from build123d import *

# Parameters (mm, degrees)
SKETCH1_W           = 103
SKETCH1_H           = 83.25
BOSS_EXTRUDE1_DEPTH = 20.2438
CUT_EXTRUDE1_DEPTH  = 17.2438
SKETCH3_W           = 15
SKETCH3_H           = 17.2438
SKETCH3_W_2         = 11
CUT_EXTRUDE2_DEPTH  = 14.9225
CUT_EXTRUDE3_DEPTH  = 2.4
SKETCH5_W           = 30
SKETCH5_H           = 6
BOSS_EXTRUDE2_DEPTH = 12.7
SKETCH6_W           = 30
SKETCH6_H           = 6
BOSS_EXTRUDE3_DEPTH = 12.7
FILLET1_R           = 4
FILLET2_R           = 0.5
FILLET3_R           = 2
FILLET4_R           = 4
FILLET5_R           = 2
SKETCH7_R           = 1.7145
CUT_EXTRUDE4_DEPTH  = 152.66642324
SKETCH8_R           = 3.81
CUT_EXTRUDE5_DEPTH  = 3.302
SKETCH11_R          = 2.38125
CUT_EXTRUDE7_DEPTH  = 151.98270874
CUT_EXTRUDE8_START  = -1
SKETCH12_R          = 4.699
CUT_EXTRUDE8_DEPTH  = 152.98270874


with BuildPart() as part:
    # Sketch1 → Boss-Extrude1 (new body)
    with BuildSketch(Plane(origin=(0, 0, 0), x_dir=(1, 0, 0), z_dir=(0, 1, 0))):
        with Locations((51.5, 41.625)):
            Rectangle(SKETCH1_W, SKETCH1_H)
    extrude(amount=BOSS_EXTRUDE1_DEPTH)

    # Sketch2 → Cut-Extrude1 (cut)
    with BuildSketch(Plane(origin=(0, 20.2438, 0), x_dir=(1, 0, 0), z_dir=(0, 1, 0))):
        Polygon((31.1, 79.75), (45.1, 79.75), (46.6, 81.25), (83.5, 81.25), (85, 79.75), (88.5, 79.75), (88.5, 11), (31.1, 11), align=None)
    extrude(amount=-CUT_EXTRUDE1_DEPTH, mode=Mode.SUBTRACT)

    # Sketch3 → Cut-Extrude2 (cut)
    with BuildSketch(Plane.XY):
        with Locations((48.5, 11.6219)):
            Rectangle(SKETCH3_W, SKETCH3_H)
        with Locations((78.5, 11.6219)):
            Rectangle(SKETCH3_W_2, SKETCH3_H)
    extrude(amount=-CUT_EXTRUDE2_DEPTH, mode=Mode.SUBTRACT)

    # Sketch4 → Cut-Extrude3 (cut)
    with BuildSketch(Plane(origin=(0, 20.2438, 0), x_dir=(1, 0, 0), z_dir=(0, 1, 0))):
        Polygon((9.5, 81.25), (101, 81.25), (101, 2), (92, 2), (92, 11), (84, 11), (84, 2), (2, 2), (2, 72.25), (9.5, 72.25), align=None)
    extrude(amount=-CUT_EXTRUDE3_DEPTH, mode=Mode.SUBTRACT)

    # Sketch5 → Boss-Extrude2 (add)
    with BuildSketch(Plane.ZY):
        with Locations((-41, 3)):
            Rectangle(SKETCH5_W, SKETCH5_H)
    boss_extrude2 = extrude(amount=BOSS_EXTRUDE2_DEPTH)

    # Mirror1: Boss-Extrude2 across plane
    add(boss_extrude2.mirror(Plane.ZY.offset(-51.5)))

    # Sketch6 → Boss-Extrude3 (add)
    with BuildSketch(Plane(origin=(0, 0, -83.25), x_dir=(-1, 0, 0), z_dir=(0, 0, -1))):
        with Locations((-51.5, 3)):
            Rectangle(SKETCH6_W, SKETCH6_H)
    extrude(amount=BOSS_EXTRUDE3_DEPTH)

    # Fillet1
    fillet1_edges = [part.edges().sort_by_distance(p)[0] for p in [
        (0, 10.1219, -83.25),
        (103, 10.1219, -83.25),
        (103, 10.1219, 0),
        (0, 10.1219, 0),
    ]]
    fillet(fillet1_edges, radius=FILLET1_R)

    # Fillet2
    fillet2_edges = [part.edges().sort_by_distance(p)[0] for p in [
        (9.5, 19.0438, -81.25),
        (92, 19.0438, -11),
        (73, 19.0438, -2),
        (41, 19.0438, -2),
        (92, 19.0438, -2),
        (2, 19.0438, -72.25),
        (9.5, 19.0438, -72.25),
        (88.5, 10.4219, -11),
        (88.5, 10.4219, -79.75),
        (31.1, 10.4219, -79.75),
        (31.1, 10.4219, -11),
        (84, 11.6219, -11),
        (56, 10.4219, -11),
        (41, 11.6219, 0),
        (56, 11.6219, 0),
        (73, 11.6219, 0),
        (84, 11.6219, 0),
        (56, 19.0438, -2),
        (41, 10.4219, -11),
        (73, 10.4219, -11),
    ]]
    fillet(fillet2_edges, radius=FILLET2_R)

    # Fillet3
    fillet3_edges = [part.edges().sort_by_distance(p)[0] for p in [
        (101, 19.0438, -2),
        (2, 19.0438, -2),
        (101, 19.0438, -81.25),
    ]]
    fillet(fillet3_edges, radius=FILLET3_R)

    # Fillet4
    fillet4_edges = [part.edges().sort_by_distance(p)[0] for p in [
        (0, 6, -41),
        (-12.7, 3, -56),
        (-12.7, 3, -26),
        (115.7, 3, -56),
        (115.7, 3, -26),
        (103, 6, -41),
        (51.5, 6, -83.25),
        (66.5, 3, -95.95),
        (36.5, 3, -95.95),
    ]]
    fillet(fillet4_edges, radius=FILLET4_R)

    # Fillet5
    fillet5_edges = [part.edges().sort_by_distance(p)[0] for p in [
        (85, 10.4219, -79.75),
        (83.5, 10.4219, -81.25),
        (46.6, 10.4219, -81.25),
        (45.1, 10.4219, -79.75),
    ]]
    fillet(fillet5_edges, radius=FILLET5_R)

    # Sketch7 → Cut-Extrude4 (cut, through all)
    with BuildSketch(Plane(origin=(0, 20.2438, 0), x_dir=(1, 0, 0), z_dir=(0, 1, 0))):
        with Locations(Location((6.35, 75.3125, 0), (0, 0, 270))):
            Circle(SKETCH7_R)
        with Locations(Location((88.265, 8.0025, 0), (0, 0, 270))):
            Circle(SKETCH7_R)
    extrude(amount=-CUT_EXTRUDE4_DEPTH, mode=Mode.SUBTRACT)

    # Sketch8 → Cut-Extrude5 (cut)
    with BuildSketch(Plane.XZ):
        with Locations(Location((6.35, -75.3125, 0), (0, 0, 270))):
            Circle(SKETCH8_R)
        with Locations(Location((88.265, -8.0025, 0), (0, 0, 270))):
            Circle(SKETCH8_R)
    extrude(amount=-CUT_EXTRUDE5_DEPTH, mode=Mode.SUBTRACT)

    # Sketch11 → Cut-Extrude7 (cut, through all)
    with BuildSketch(Plane(origin=(0, 6, 0), x_dir=(1, 0, 0), z_dir=(0, 1, 0))):
        with Locations(Location((-6.35, 41, 0), (0, 0, 270))):
            Circle(SKETCH11_R)
    cut_extrude7 = extrude(amount=-CUT_EXTRUDE7_DEPTH, mode=Mode.SUBTRACT)

    # Sketch12 → Cut-Extrude8 (cut)
    with BuildSketch(Plane(origin=(0, 6, 0), x_dir=(1, 0, 0), z_dir=(0, 1, 0)).offset(CUT_EXTRUDE8_START)):
        with Locations(Location((-6.35, 41, 0), (0, 0, 59.992960011))):
            Circle(SKETCH12_R)
    cut_extrude8 = extrude(amount=CUT_EXTRUDE8_DEPTH, mode=Mode.SUBTRACT)

    # Sketch-Pattern2: Cut-Extrude7, Cut-Extrude8 at 2 more places
    with Locations((57.85, 0, -48.6), (115.7, 0, 0)):
        add(cut_extrude7, mode=Mode.SUBTRACT)
        add(cut_extrude8, mode=Mode.SUBTRACT)


solid = part.part
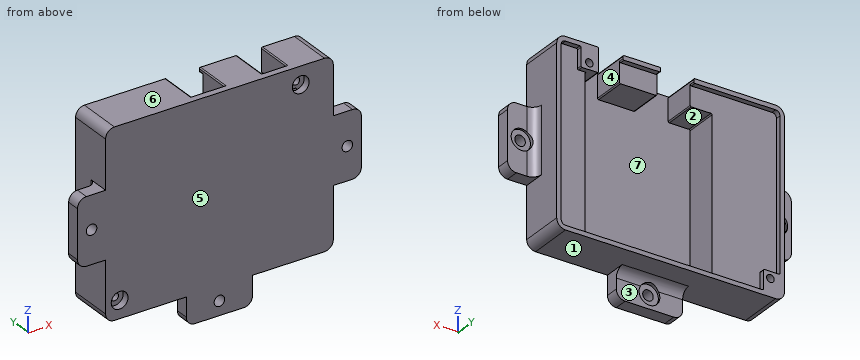
Here's how the part is built. I have some questions about the finished solid (model axes, mm). Face numbers are marked on the shaded views. A direction names the side the tool comes from. Give positions to 0.01 mm unless a question says otherwise; leave off trailing zeros. Loops run counter-clockwise (first coordinate to the right, second up) from the corner with the lowest first, then second, coordinate; pieces in that order, holes last. Notation, with made-up numbers: (27.25, 28.5) -> (71.25, 28.5) arc R28 ccw to (71.25, 66.5) -> close; hole circle Ø9 at (85.25, 30). An arc over 180 degrees is marked (long way). Answer as a JSON object with one key per item and string values. Group by question number.
Item 1: On a 3-axis mill with a long thin cutter (end or side, diameter ignored), from which of +Z, -Z, +X, -X, +Y, -Y can I reach the whole of each face in a straight line? I mean the marked faces 1, 2, 3 and 4. Say none if no direction works.
Item 2: Will these pins go through, and if not, where does the flat tip stop? pin 1 (7.5 mm diameter, centred on x = 110.5, z = -43, fed in from +Y); pin 2 (10 mm diameter, centred on y = 2.5, z = -68.5, fed in from +X); pin 3 (4 mm diameter, centred on x = 6.35, z = -75.31, fed in from -Y).
Item 3: Imagine slicing it at D-D on x = 34. Write out the boundary of the cut face in (y, z), then the cut area to 3 significant figures.
Item 4: Imagine slicing it at B-B on z = -89.6. Write out the boundary of the cut face in (x, y), then the cut area to 3 significant figures.
Item 5: Imagine slicing it at C-C on z = -41. Give the number of separate pieces and of enclosed holes in the cut face, then the cut area to 3 significant figures.
Item 6: I need wall thicknesses on L1, parallel to X at y = 11.75, z = -10; L2, parallel to X at y = 5.6, z = -41; L3, parallel to Z at x = 40, y = 17. Which ranges of each line are inside material? Lowest first, please.
Item 7: Thinking about a two-plate mould opening in Z: for the marked faces 5, 6 and 7, which applies, pulls with the +Z half, pulls with the -Z half, needs draft (parallel to the pull), parting line crosses it, or undercut?
Item 8: Imagine slicing it at A-A on x = 51.5. Write out the boundary of the cut face in (y, z).
Answer list:
{
 "1": {"face 1": "-Z, +Y", "face 2": "+Y", "face 3": "-Z, +X, -X, +Y", "face 4": "+Z, +Y"},
 "2": {"pin 1": "stops at y = 6", "pin 2": "stops at x = 103", "pin 3": "stops at y = 3.3"},
 "3": {"outline": "(0, -83.25) -> (20.24, -83.25) -> (20.24, -81.25) -> (17.84, -81.25) -> (17.84, -79.75) -> (3, -79.75) -> (3, -11) -> (17.84, -11) -> (17.84, -2) -> (20.24, -2) -> (20.24, 0) -> (0, 0) -> close", "area": "475 mm2"},
 "4": {"outline": "(36.5, 0) -> (49.12, 0) -> (49.12, 5) -> (46.8, 5) -> (46.8, 6) -> (36.5, 6) -> close; (53.88, 0) -> (66.5, 0) -> (66.5, 6) -> (56.2, 6) -> (56.2, 5) -> (53.88, 5) -> close", "area": "147 mm2"},
 "5": {"separate pieces": "3", "enclosed holes": "0", "area": "1,090 mm2"},
 "6": {"L1": "x = 0 to 41, 56 to 73, 84 to 103", "L2": "x = -12.7 to -11.05, -1.65 to 31.1, 88.5 to 104.65, 114.05 to 115.7", "L3": "z = -83.25 to -79.75, -11 to 0"},
 "7": {"face 5": "needs draft", "face 6": "pulls with the +Z half", "face 7": "undercut"},
 "8": {"outline": "(0, -95.95) -> (6, -95.95) -> (6, -94.3) -> (5, -94.3) -> (5, -91.98) -> (0, -91.98) -> close; (0, -87.22) -> (5, -87.22) -> (5, -84.9) -> (6.76, -84.9) arc R4 cw to (10, -83.25) -> (20.24, -83.25) -> (20.24, -81.25) -> (3, -81.25) -> (3, 0) -> (0, 0) -> close"}
}
